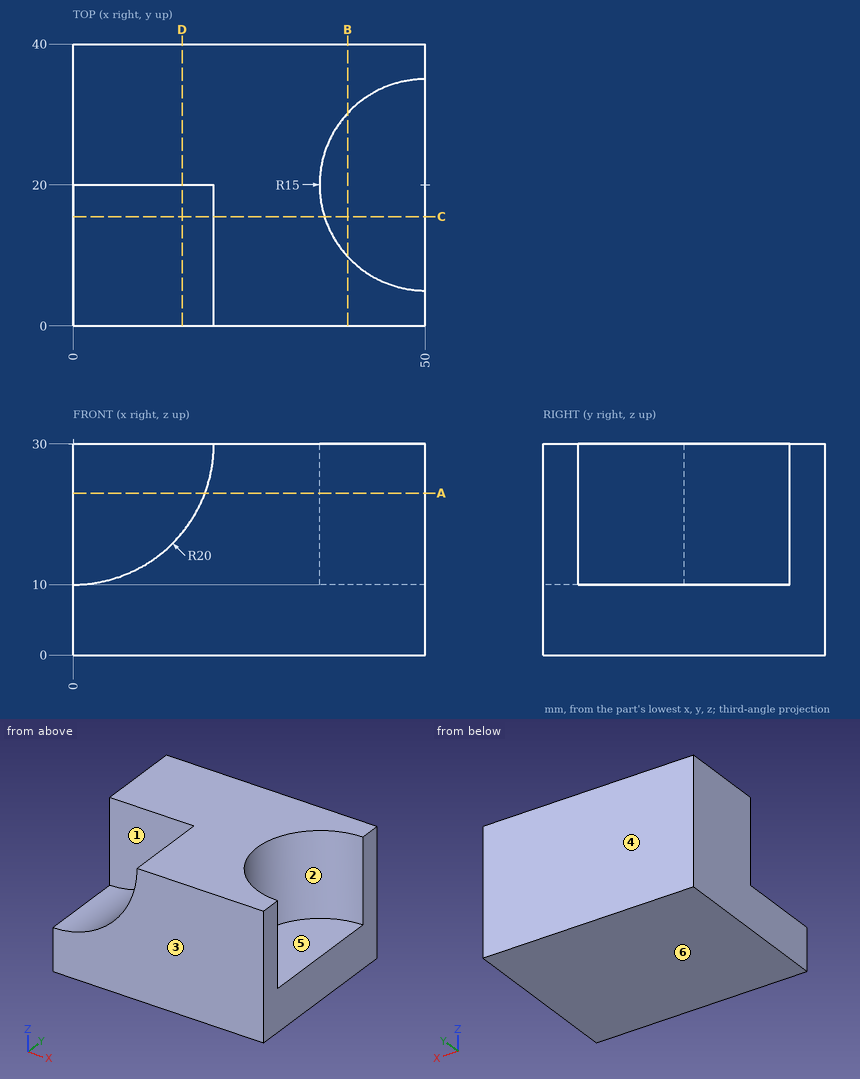
Can you work these out from the drawing? Everything is in mm from the part's minimum corner. A direction names the side the tool comes from. Coordinates: 2 decimals unless noted, no trailing zeros. Loops run counter-clockwise (first coordinate to the right, second up) from the corner with the lowest first, then second, coordinate; pieces in that order, holes last. Notation, with made-up numbers: (-15, 48.5) -> (40, 48.5) arc R23 cw to (40, 60.5) -> close; hole circle Ø5 at (24, 54). An arc over 180 degrees is marked (long way). Return JSON: item names as keys, results as strings.
1) Thinking about a two-plate mould opening in Y: for the marked faces 4, 5 and 6, which applies, +Y half, -Y half, draft (parallel to the pull), parting line (faces both ways), or undercut?
Results below:
{"face 4": "+Y half", "face 5": "undercut", "face 6": "draft"}
2) For the marked faces 1, 2 and 3, which set-ups out of +Z, -Z, +X, -X, +Y, -Y let a thin tool reach every point of the face, with its end or its side?
Results below:
{"face 1": "+Z, -X, -Y", "face 2": "+Z, +X", "face 3": "+Z, -Z, +X, -X, -Y"}
3) If we section it at A-A, the plane z = 23: Write out the boundary of the cut face in (x, y) (3 decimals).
Results below:
{"outline": "(0, 20) -> (18.735, 20) -> (18.735, 0) -> (50, 0) -> (50, 5) arc R15 cw to (50, 35) -> (50, 40) -> (0, 40) -> close"}
4) Will these pins go through, and if not, where does the flat tip stop? pin 1 (12 mm diameter, centred on x = 44.5, y = 27.5, fed in from +Z); pin 2 (2 mm diameter, centred on y = 22, z = 21.5, fed in from +X).
Results below:
{"pin 1": "z = 30", "pin 2": "x = 35.3"}
5) If we section it at C-C, the plane y = 15.5: Write out the boundary of the cut face in (x, z), then the cut area to 3 significant figures.
Results below:
{"outline": "(0, 0) -> (50, 0) -> (50, 10) -> (35.69, 10) -> (35.69, 30) -> (20, 30) arc R20 cw to (0, 10) -> close", "area": "900 mm²"}
6) If we section it at D-D, the plane x = 15.5: Write out the boundary of the cut face in (y, z), then the cut area to 3 significant figures.
Results below:
{"outline": "(0, 0) -> (40, 0) -> (40, 30) -> (20, 30) -> (20, 17.36) -> (0, 17.36) -> close", "area": "947 mm²"}
7) If we section it at B-B, the plane x = 39: Write out the boundary of the cut face in (y, z), then the cut area to 3 significant figures.
Results below:
{"outline": "(0, 0) -> (40, 0) -> (40, 30) -> (30.2, 30) -> (30.2, 10) -> (9.8, 10) -> (9.8, 30) -> (0, 30) -> close", "area": "792 mm²"}
8) I need wall thicknesses on line 1 (Y direction, x = 10, z = 23.25); line 2 (Z direction, x = 40.5, y = 11.5); line 3 (Y direction, x = 38, z = 14.5). Which ranges of each line are inside material? Lowest first, please. Write a range as from..to.
Results below:
{"line 1": "20..40", "line 2": "0..10", "line 3": "0..11, 29..40"}
